```python
from build123d import *

# Parameters (mm, degrees)
BOSS_EXTRUDE1_DEPTH = 19.05
SKETCH2_R           = 3.556
CUT_EXTRUDE1_DEPTH  = 5.08
CUT_EXTRUDE2_REACH  = 15.638
SKETCH2_3_R         = 3.556


with BuildPart() as part:
    # Sketch1 → Boss-Extrude1 (new body)
    with BuildSketch(Plane(origin=(0, 0, 0), x_dir=(1, 0, 0), z_dir=(0, 1, 0))):
        with BuildLine():
            ThreePointArc((77.47, 122.910544885), (68.991544122, 127.862307909), (60.198, 132.230116615))
            Line((60.198, 132.230116615), (60.198, 118.592544885))
            Line((60.198, 118.592544885), (77.47, 118.592544885))
            Line((77.47, 118.592544885), (77.47, 122.910544885))
        make_face()
    extrude(amount=BOSS_EXTRUDE1_DEPTH)

    # Sketch2 → Cut-Extrude1 (cut)
    with BuildSketch(Plane.XY.offset(-118.592544885)):
        with Locations((67.945, 9.525)):
            Circle(SKETCH2_R)
        Polygon((64.535457985, 3.6195), (71.354542015, 3.6195), (74.764084029, 9.525), (71.354542015, 15.4305), (64.535457985, 15.4305), (61.125915971, 9.525), align=None)
        with Locations((67.945, 9.525)):
            Circle(SKETCH2_R, mode=Mode.SUBTRACT)
    extrude(amount=-CUT_EXTRUDE1_DEPTH, mode=Mode.SUBTRACT)

    # Sketch2_3 → Cut-Extrude2 (cut, up to next)
    with BuildSketch(Plane.XY.offset(-118.592544885), mode=Mode.PRIVATE) as cut_extrude2_sk1:
        with Locations((67.945, 9.525)):
            Circle(SKETCH2_3_R)
    cut_extrude2_tool1 = extrude(cut_extrude2_sk1.sketch, amount=-CUT_EXTRUDE2_REACH, mode=Mode.PRIVATE) & part.part
    add(cut_extrude2_tool1.solids().sort_by_distance((67.945, 9.525, -118.592545))[0], mode=Mode.SUBTRACT)


solid = part.part
```
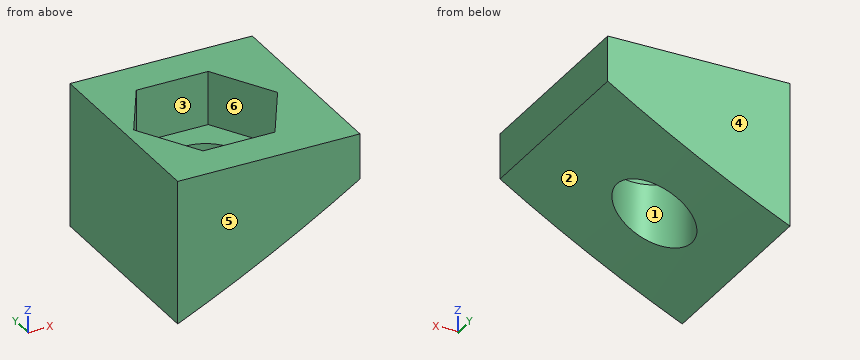
The listing builds one solid part. Answer for the finished solid, in the listing's coordinates (mm). Face numbers are marked on the shaded views. A direction names the side the tool comes from. Give positions to 0.01 mm unless a question says otherwise; leave off trailing zeros. Write each loop counter-clockwise with the first axis right and the second up, starting at its lowest first coordinate (ties: lowest second). Pieces come first, ordered by that corner, then holes. Notation, with made-up numbers: (-29.5, 24.25) - (-4.5, 24.25) arc R30 cw to (-4.5, 58.25) - close; hole circle Ø10 at (3.25, 31). An arc over 180 degrees is marked (long way). Use one line per item in the form item = value. Start each with the question number.
1) The mould has two halves that part along X. Classify the marked faces 1, 2, 3 and 4: pulls with the +X half, pulls with the -X half, needs draft (parallel to the pull), parting line crosses it, or undercut.
2) Find section B-B on x = 65. Determine the outline of the cut face in (y, z), plus the area to 3 significant figures.
3) Consider line 1 along Y through (x, z) = (65.75, -120.5); line 2 along X through (y, z) = (12, -123.75); line 3 along Y through (x, z) = (73.75, -123.5). Determine where each line is inside the solid, lowest interval first. Write a range as from..to.
4) Find section D-D on y = 17. Determine the outline of the cut face in (x, z).
5) A tool of negligible diameter and unlimited length cuts with its end or side. For the marked faces 5 and 6, from which of +Z, -Z, +X, -X, +Y, -Y can it reach the whole face along a straight path? Write none if from no direction.
6) Find section C-C on y = 7. Determine the outline of the cut face in (x, z).
7) Flat-ended cylindrical pins translate along their axes: pin 1 Ø1.5 at (x, y) = (68, 11.5) entering from -Z; pin 2 Ø9 at (x, y) = (67.945, 9.525) entering from -Z; pin 3 Ø10 at (x, y) = (62.5, 8.5) entering from -Z; pin 4 Ø6 at (x, y) = (73, 2.5) entering from -Z. Find the tip coordinate at first contact, or state that the pin passes through.
Geometry results:
q1.face_1 = undercut
q1.face_2 = pulls with the +X half
q1.face_3 = undercut
q1.face_4 = needs draft
q2.outline = (0, -129.94) - (7.53, -129.94) - (7.53, -123.67) - (3.62, -123.67) - (3.62, -118.59) - (0, -118.59) - close; (11.52, -129.94) - (19.05, -129.94) - (19.05, -118.59) - (15.43, -118.59) - (15.43, -123.67) - (11.52, -123.67) - close
q2.area = 131 mm2
q3.line_1 = 0..3.62, 15.43..19.05
q3.line_2 = 60.2..65.39, 70.5..76.12
q3.line_3 = 0..7.77, 11.28..19.05
q4.outline = (60.2, -132.23) arc R145.29 ccw to (77.47, -122.91) - (77.47, -118.59) - (60.2, -118.59) - close
q5.face_5 = +Z, -Z, +X, -X, -Y
q5.face_6 = +Z
q6.outline = (60.2, -132.23) arc R145.29 ccw to (65.44, -129.72) - (65.44, -123.67) - (62.58, -123.67) - (62.58, -118.59) - (60.2, -118.59) - close; (70.45, -127.07) arc R145.29 ccw to (77.47, -122.91) - (77.47, -118.59) - (73.31, -118.59) - (73.31, -123.67) - (70.45, -123.67) - close
q7.pin_1 = through
q7.pin_2 = -130.7
q7.pin_3 = -132.23
q7.pin_4 = -127.31
